```python
from build123d import *

# Parameters (mm, degrees)
BOSS_EXTRUDE1_DEPTH = 10
SKETCH3_R           = 19.075
CUT_EXTRUDE1_DEPTH  = 11
SKETCH4_W           = 1.877089928
SKETCH4_H           = 9.959436021
CUT_EXTRUDE2_DEPTH  = 11
SKETCH5_R           = 1.59
CUT_EXTRUDE3_DEPTH  = 10
SKETCH6_R           = 1.59
CUT_EXTRUDE4_DEPTH  = 10
SKETCH7_W           = 10
SKETCH7_H           = 1
CUT_EXTRUDE5_DEPTH  = 29.718


with BuildPart() as part:
    # Sketch2 → Boss-Extrude1 (new body)
    with BuildSketch(Plane.XY):
        with BuildLine():
            Line((14.400910076, -32.666118303), (-14.400910076, -32.666118303))
            Line((-14.400910076, -32.666118303), (-14.400910076, -29.486118303))
            Line((-14.400910076, -29.486118303), (-3.18, -29.486118303))
            Line((-3.18, -29.486118303), (-3.18, -23.727857046))
            ThreePointArc((-3.18, -23.727857046), (-23.94, 0), (-3.18, 23.727857046))
            Line((-3.18, 23.727857046), (-3.18, 29.011332471))
            Line((-3.18, 29.011332471), (3.18, 29.011332471))
            Line((3.18, 29.011332471), (3.18, 23.727857046))
            ThreePointArc((3.18, 23.727857046), (23.939582665, -0.141357095), (2.89957421, -23.763755372))
            Line((2.89957421, -23.763755372), (2.89957421, -29.486118303))
            Line((2.89957421, -29.486118303), (14.400910076, -29.486118303))
            Line((14.400910076, -29.486118303), (14.400910076, -32.666118303))
        make_face()
    extrude(amount=BOSS_EXTRUDE1_DEPTH)

    # Sketch3 → Cut-Extrude1 (cut, through all)
    with BuildSketch(Plane.XY.offset(10)):
        Circle(SKETCH3_R)
    extrude(amount=-CUT_EXTRUDE1_DEPTH, mode=Mode.SUBTRACT)

    # Sketch4 → Cut-Extrude2 (cut, through all)
    with BuildSketch(Plane.XY.offset(10)):
        with Locations((0, 24.031614461)):
            Rectangle(SKETCH4_W, SKETCH4_H)
    extrude(amount=-CUT_EXTRUDE2_DEPTH, mode=Mode.SUBTRACT)

    # Sketch5 → Cut-Extrude3 (cut)
    with BuildSketch(Plane(origin=(3.18, 0, 0), x_dir=(0, 0, -1), z_dir=(1, 0, 0))):
        with Locations((-5, 26.369594759)):
            Circle(SKETCH5_R)
    extrude(amount=-CUT_EXTRUDE3_DEPTH, mode=Mode.SUBTRACT)

    # Sketch6 → Cut-Extrude4 (cut)
    with BuildSketch(Plane(origin=(0, -29.486118303, 0), x_dir=(1, 0, 0), z_dir=(0, 1, 0))):
        with Locations((8.912608952, -5.289784221)):
            Circle(SKETCH6_R)
        with Locations((-8.273500585, -5.289784221)):
            Circle(SKETCH6_R)
    extrude(amount=-CUT_EXTRUDE4_DEPTH, mode=Mode.SUBTRACT)

    # Sketch7 → Cut-Extrude5 (cut)
    with BuildSketch(Plane(origin=(3.18, 0, 0), x_dir=(0, 0, -1), z_dir=(1, 0, 0))):
        with Locations((-5, 23.227857046)):
            Rectangle(SKETCH7_W, SKETCH7_H)
    extrude(amount=CUT_EXTRUDE5_DEPTH, mode=Mode.SUBTRACT)


solid = part.part
```
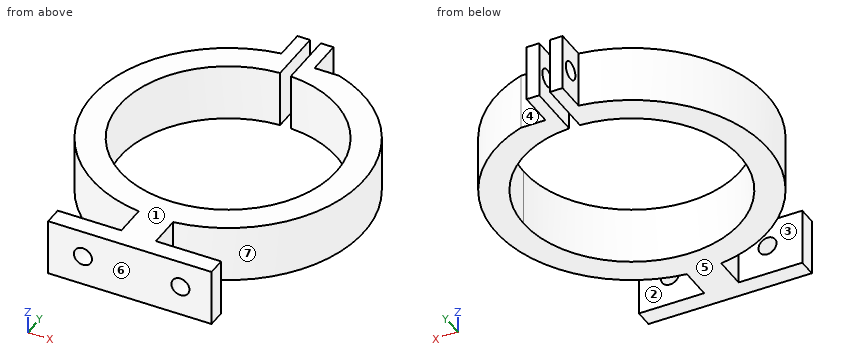
Geometry: final body of the model. Coordinates: model frame, mm. Face numbers are marked on the shaded views. A direction names the side the tool comes from. Round coordinates to 2 decimals unless told otherwise and drop trailing zeros. Order: outer loops, then holes, each group sorted by start corner. A loop starts at its lowest first (then second) coordinate and runs counter-clockwise, first axis right, second up. Notation, with made-up numbers: (58, -10) -> (68, -10) arc R23 cw to (68, 3) -> close; hole circle Ø3 at (59, 80). An arc over 180 degrees is marked (long way). Use one line per item in the form item = value.
(1) First-contact query: pin 1 Ø2.5 at (y, z) = (-31.5, 5.5) entering from +X; pin 2 Ø5 at (y, z) = (25.5, 2.5) entering from +X; pin 3 Ø2.5 at (x, z) = (8.91, 5.29) entering from +Y; pin 4 Ø5 at (x, z) = (-8.27, 5.29) entering from -Y. Flat tips, straight axial feed; report the tip coordinate or a pass-through.
Results list:
pin_1 = 14.4
pin_2 = 3.18
pin_3 = 22.68
pin_4 = -32.67
(2) Access query for the marked faces 1, 2 and 3. Directions: +Z, -Z, +X, -X, +Y, -Y. A direction counts if a zero-diameter tool reaches every point of the face in a straight line with its end or side. Return the directions, or none.
Results list:
face_1 = +Z, +X, -X, +Y, -Y
face_2 = +Z, -Z, +X
face_3 = +Z, -Z, -X
(3) Section A-A on x = -12. Return loops of the section in (y, z), and give its area (3 significant figures).
Results list:
outline = (-32.67, 0) -> (-29.49, 0) -> (-29.49, 10) -> (-32.67, 10) -> close; (-20.72, 0) -> (-14.83, 0) -> (-14.83, 10) -> (-20.72, 10) -> close; (14.83, 0) -> (20.72, 0) -> (20.72, 10) -> (14.83, 10) -> close
area = 150 mm^2
(4) Section C-C on z = 8.5. Return loops of the section in (x, y) (3 decimals), and give its area (3 significant figures).
Results list:
outline = (-14.401, -32.666) -> (14.401, -32.666) -> (14.401, -29.486) -> (2.9, -29.486) -> (2.9, -23.764) arc R23.94 ccw to (7.521, 22.728) -> (3.18, 22.728) -> (3.18, 29.011) -> (0.939, 29.011) -> (0.939, 19.052) arc R19.075 cw (long way) to (-0.939, 19.052) -> (-0.939, 29.011) -> (-3.18, 29.011) -> (-3.18, 23.728) arc R23.94 ccw to (-3.18, -23.728) -> (-3.18, -29.486) -> (-14.401, -29.486) -> close
area = 795 mm^2
(5) Draft query along Y for the marked faces 4, 5, 6 and 7. Return one class per face: pulls with the +Y half, pulls with the -Y half, needs draft (parallel to the pull), parting line crosses it, or undercut.
Results list:
face_4 = pulls with the +Y half
face_5 = needs draft
face_6 = pulls with the -Y half
face_7 = undercut
(6) Section D-D on x = 18. Return loops of the section in (y, z), and give its area (3 significant figures).
Results list:
outline = (-15.78, 0) -> (-6.31, 0) -> (-6.31, 10) -> (-15.78, 10) -> close; (6.31, 0) -> (15.78, 0) -> (15.78, 10) -> (6.31, 10) -> close
area = 189 mm^2
(7) Ray query, probe 1 along Y at (x, z) = (2.1, 5); probe 2 along X at (y, z) = (-30, 6.5); probe 3 along Y at (x, z) = (8, 8.75). Return the intervals inside material, ascending. Write a range as [from, to].
Results list:
probe_1 = [-32.67, -18.96], [18.96, 24.78], [27.96, 29.01]
probe_2 = [-14.4, -9.3], [-7.24, 7.88], [9.94, 14.4]
probe_3 = [-32.67, -29.49], [-22.56, -17.32], [17.32, 22.56]
(8) Section B-B on y = 15.5. Return loops of the section in (x, z).
Results list:
outline = (-18.24, 0) -> (-11.12, 0) -> (-11.12, 10) -> (-18.24, 10) -> close; (11.12, 0) -> (18.24, 0) -> (18.24, 10) -> (11.12, 10) -> close
